Work out the finished part from the listing and answer in its coordinate system (mm). Coordinates: 2 decimals unless noted, no trailing zeros. Write item = value, one per line. Start each with the question number.
Q1. Flat-ended cylindrical pins translate along their axes: pin 1 (5 mm diameter, centred on x = 16.03, z = 0.36, fed in from +Y); pin 2 (5 mm diameter, centred on x = 34.03, z = 28.86, fed in from +Y). Find the tip coordinate at first contact, or state that the pin passes through.
Q2. Straight lines are drawn through the part: L1, parallel to Z at x = 34.5, y = 2.5; L2, parallel to X at y = 9.75, z = 0; L3, parallel to Z at x = -26.5, y = 7.5. For each, find the intervals that lie inside material, in ascending order. Write a range as from..to.
Q3. The part is cut by section A-A, the plane y = 3.25. Count the separate pieces of the cut face and the enclosed holes in it, plus the area to 3 significant figures.
Q4. For a pull along Z with two mould halves and no side action, classify faces 1 (the flat face through (-4, 5, -2.641)), 2 (the flat face through (-70.97, 5, 17)), 3 (the cylindrical face through (56.1, 4.93, 28.21)) as +Z half, -Z half, draft (parallel to the pull), parting line (faces both ways), or undercut.
```python
from build123d import *

# Parameters (mm, degrees)
SKETCH1_W           = 136
SKETCH1_H           = 38
SKETCH1_R           = 1.5
SKETCH1_R_2         = 3
BOSS_EXTRUDE1_DEPTH = 10


with BuildPart() as part:
    # Sketch1 → Boss-Extrude1 (new body)
    with BuildSketch(Plane(origin=(0, 0, 0), x_dir=(1, 0, 0), z_dir=(0, 1, 0))):
        with Locations((-2.969502184, -16.359463259)):
            Rectangle(SKETCH1_W, SKETCH1_H)
        with Locations(Location((-15.969502184, -0.359463259, 0), (0, 0, 270))):
            Circle(SKETCH1_R, mode=Mode.SUBTRACT)
        with Locations(Location((16.030497816, -0.359463259, 0), (0, 0, 270))):
            Circle(SKETCH1_R, mode=Mode.SUBTRACT)
        with Locations(Location((16.030497816, -32.359463259, 0), (0, 0, 270))):
            Circle(SKETCH1_R, mode=Mode.SUBTRACT)
        with Locations(Location((-15.969502184, -32.359463259, 0), (0, 0, 270))):
            Circle(SKETCH1_R, mode=Mode.SUBTRACT)
        with Locations(Location((-65.969502184, -3.859463259, 0), (0, 0, 270))):
            Circle(SKETCH1_R_2, mode=Mode.SUBTRACT)
        with Locations(Location((-40.969502184, -3.859463259, 0), (0, 0, 270))):
            Circle(SKETCH1_R_2, mode=Mode.SUBTRACT)
        with Locations(Location((-40.969502184, -28.859463259, 0), (0, 0, 270))):
            Circle(SKETCH1_R_2, mode=Mode.SUBTRACT)
        with Locations(Location((-65.969502184, -28.859463259, 0), (0, 0, 270))):
            Circle(SKETCH1_R_2, mode=Mode.SUBTRACT)
        with Locations(Location((-28.469502184, -28.859463259, 0), (0, 0, 270))):
            Circle(SKETCH1_R_2, mode=Mode.SUBTRACT)
        with Locations(Location((-53.469502184, -3.859463259, 0), (0, 0, 270))):
            Circle(SKETCH1_R_2, mode=Mode.SUBTRACT)
        with Locations(Location((-53.469502184, -28.859463259, 0), (0, 0, 270))):
            Circle(SKETCH1_R_2, mode=Mode.SUBTRACT)
        with Locations(Location((-28.469502184, -3.859463259, 0), (0, 0, 270))):
            Circle(SKETCH1_R_2, mode=Mode.SUBTRACT)
        with Locations(Location((34.030497816, -3.859463259, 0), (0, 0, 270))):
            Circle(SKETCH1_R_2, mode=Mode.SUBTRACT)
        with Locations(Location((59.030497816, -28.859463259, 0), (0, 0, 270))):
            Circle(SKETCH1_R_2, mode=Mode.SUBTRACT)
        with Locations(Location((59.030497816, -3.859463259, 0), (0, 0, 270))):
            Circle(SKETCH1_R_2, mode=Mode.SUBTRACT)
        with Locations(Location((34.030497816, -28.859463259, 0), (0, 0, 270))):
            Circle(SKETCH1_R_2, mode=Mode.SUBTRACT)
        with Locations(Location((21.530497816, -28.859463259, 0), (0, 0, 270))):
            Circle(SKETCH1_R_2, mode=Mode.SUBTRACT)
        with Locations(Location((46.530497816, -28.859463259, 0), (0, 0, 270))):
            Circle(SKETCH1_R_2, mode=Mode.SUBTRACT)
        with Locations(Location((21.530497816, -3.859463259, 0), (0, 0, 270))):
            Circle(SKETCH1_R_2, mode=Mode.SUBTRACT)
        with Locations(Location((46.530497816, -3.859463259, 0), (0, 0, 270))):
            Circle(SKETCH1_R_2, mode=Mode.SUBTRACT)
    extrude(amount=BOSS_EXTRUDE1_DEPTH)


solid = part.part
```
Model answer:
q1.pin_1 = 10
q1.pin_2 = through
q2.L1 = -2.64..0.9, 6.82..25.9, 31.82..35.36
q2.L2 = -70.97..-17.43, -14.51..14.57, 17.49..65.03
q2.L3 = -2.64..1.6, 6.12..26.6, 31.12..35.36
q3.separate_pieces = 1
q3.enclosed_holes = 20
q3.area = 4,690 mm2
q4.face_1 = -Z half
q4.face_2 = draft
q4.face_3 = undercut
